Part model, mm, in its own coordinate system. A direction names the side the tool comes from. Coordinates: 2 decimals unless noted, no trailing zeros. Order: outer loops, then holes, each group sorted by start corner. A loop starts at its lowest first (then second) coordinate and runs counter-clockwise, first axis right, second up.
from build123d import *

# Parameters (mm, degrees)
CROQUIS1_R              = 20.65
CROQUIS1_R_2            = 1.5
SALIENTE_EXTRUIR1_DEPTH = 5
SALIENTE_EXTRUIR2_DEPTH = 20
CROQUIS3_R              = 1.5
CORTAR_EXTRUIR1_DEPTH   = 20
CROQUIS4_R              = 2
CORTAR_EXTRUIR2_DEPTH   = 166.327956902
CHAFL_N1_SIZE           = 15
CROQUIS5_R              = 7
CROQUIS5_R_2            = 2
CORTAR_EXTRUIR3_DEPTH   = 30
CORTAR_EXTRUIR4_START   = 30
CROQUIS6_R              = 6.5
CROQUIS6_R_2            = 1.5
CORTAR_EXTRUIR4_DEPTH   = 30


with BuildPart() as part:
    # Croquis1 → Saliente-Extruir1 (new, symmetric)
    with BuildSketch(Plane(origin=(0, 0, 0), x_dir=(0, 0, -1), z_dir=(1, 0, 0))):
        with BuildLine():
            Line((-109.696551146, -120), (109.696551146, -120))
            Line((109.696551146, -120), (30.310889132, 17.5))
            ThreePointArc((30.310889132, 17.5), (0, 35), (-30.310889132, 17.5))
            Line((-30.310889132, 17.5), (-109.696551146, -120))
        make_face()
        Circle(CROQUIS1_R, mode=Mode.SUBTRACT)
        with Locations((-30, 0)):
            Circle(CROQUIS1_R_2, mode=Mode.SUBTRACT)
        with Locations((30, 0)):
            Circle(CROQUIS1_R_2, mode=Mode.SUBTRACT)
    extrude(amount=SALIENTE_EXTRUIR1_DEPTH, both=True)

    # Croquis2 → Saliente-Extruir2 (add)
    with BuildSketch(Plane.ZY.offset(5)):
        Polygon((-109.696551146, -120), (-103.923048454, -110), (103.923048454, -110), (109.696551146, -120), align=None)
    extrude(amount=SALIENTE_EXTRUIR2_DEPTH)

    # Croquis3 → Cortar-Extruir1 (cut)
    with BuildSketch(Plane(origin=(0, -110, 0), x_dir=(1, 0, 0), z_dir=(0, 1, 0))):
        with Locations(Location((-15, 60, 0), (0, 0, 270))):
            Circle(CROQUIS3_R)
        with Locations(Location((-15, -60, 0), (0, 0, 270))):
            Circle(CROQUIS3_R)
        with Locations(Location((-15, 0, 0), (0, 0, 270))):
            Circle(CROQUIS3_R)
    extrude(amount=-CORTAR_EXTRUIR1_DEPTH, mode=Mode.SUBTRACT)

    # Croquis4 → Cortar-Extruir2 (cut, through all)
    with BuildSketch(Plane(origin=(5, 0, 0), x_dir=(0, 0, -1), z_dir=(1, 0, 0))):
        with Locations((-40, -100)):
            Circle(CROQUIS4_R)
        with Locations((40, -100)):
            Circle(CROQUIS4_R)
    extrude(amount=-CORTAR_EXTRUIR2_DEPTH, mode=Mode.SUBTRACT)

    # Chaflán1
    # the kernel refuses this chamfer: 15 mm, written as the material it adds along each edge
    with BuildSketch(Plane(origin=(-5, -110, -142.498293274), x_dir=(0.02749587661058636, 0.9996219169112966, 0), z_dir=(0, 0, 1))) as chafl_n1_piece_1_section:
        Polygon((CHAFL_N1_SIZE * 0.999621916911, CHAFL_N1_SIZE * 0.0274958766106), (-CHAFL_N1_SIZE * 0.0274958766106, CHAFL_N1_SIZE * 0.999621916911), (0, 0), align=None)
    chafl_n1_piece_1 = extrude(amount=284.996586547, mode=Mode.PRIVATE)
    chafl_n1_piece_1 = split(chafl_n1_piece_1, bisect_by=Plane(origin=(-9.982063802, -61.362690363, 75.842284643), z_dir=(0, -0.500000000000004, -0.8660254037844364)), keep=Keep.TOP, mode=Mode.PRIVATE)
    chafl_n1_piece_1 = split(chafl_n1_piece_1, bisect_by=Plane(origin=(-9.982063802, -61.362690271, -75.84228459), z_dir=(0, -0.4999999999999981, 0.8660254037844397)), keep=Keep.TOP, mode=Mode.PRIVATE)
    chafl_n1_piece_1 = chafl_n1_piece_1 - Plane(origin=(-9.982063802, -100, 40), x_dir=(0, 0, -1), z_dir=(1, 0, 0)) * Cylinder(2, 630, mode=Mode.PRIVATE)
    chafl_n1_piece_1 = chafl_n1_piece_1 - Plane(origin=(-9.982063802, -100, -40), x_dir=(0, 0, -1), z_dir=(1, 0, 0)) * Cylinder(2, 630, mode=Mode.PRIVATE)
    chafl_n1_piece_1 = chafl_n1_piece_1 - Plane(origin=(-15, -105.150253756, -60), x_dir=(0, 0, 1), z_dir=(0, 1, 0)) * Cylinder(1.5, 630, mode=Mode.PRIVATE)
    chafl_n1_piece_1 = chafl_n1_piece_1 - Plane(origin=(-15, -105.150253756, 0), x_dir=(0, 0, 1), z_dir=(0, 1, 0)) * Cylinder(1.5, 630, mode=Mode.PRIVATE)
    chafl_n1_piece_1 = chafl_n1_piece_1 - Plane(origin=(-15, -105.150253756, 60), x_dir=(0, 0, 1), z_dir=(0, 1, 0)) * Cylinder(1.5, 630, mode=Mode.PRIVATE)
    add(chafl_n1_piece_1)

    # Croquis5 → Cortar-Extruir3 (cut)
    # profile 1 of 2: a face of its own
    with BuildSketch(Plane.ZY.offset(5)):
        with Locations((-40, -100)):
            Circle(CROQUIS5_R)
        with Locations(Location((-40, -100, 0), (0, 0, 180))):
            Circle(CROQUIS5_R_2, mode=Mode.SUBTRACT)
    # profile 2 of 2: a face of its own
    with BuildSketch(Plane.ZY.offset(5)):
        with Locations((40, -100)):
            Circle(CROQUIS5_R)
        with Locations(Location((40, -100, 0), (0, 0, 180))):
            Circle(CROQUIS5_R_2, mode=Mode.SUBTRACT)
    extrude(amount=CORTAR_EXTRUIR3_DEPTH, mode=Mode.SUBTRACT)

    # Croquis6 → Cortar-Extruir4 (cut)
    # profile 1 of 3: a face of its own
    with BuildSketch(Plane(origin=(0, -110, 0), x_dir=(1, 0, 0), z_dir=(0, 1, 0)).offset(CORTAR_EXTRUIR4_START)):
        with Locations((-15, 60)):
            Circle(CROQUIS6_R)
        with Locations(Location((-15, 60, 0), (0, 0, 270))):
            Circle(CROQUIS6_R_2, mode=Mode.SUBTRACT)
    # profile 2 of 3: a face of its own
    with BuildSketch(Plane(origin=(0, -110, 0), x_dir=(1, 0, 0), z_dir=(0, 1, 0)).offset(CORTAR_EXTRUIR4_START)):
        with Locations((-15, 0)):
            Circle(CROQUIS6_R)
        with Locations(Location((-15, 0, 0), (0, 0, 270))):
            Circle(CROQUIS6_R_2, mode=Mode.SUBTRACT)
    # profile 3 of 3: a face of its own
    with BuildSketch(Plane(origin=(0, -110, 0), x_dir=(1, 0, 0), z_dir=(0, 1, 0)).offset(CORTAR_EXTRUIR4_START)):
        with Locations((-15, -60)):
            Circle(CROQUIS6_R)
        with Locations(Location((-15, -60, 0), (0, 0, 270))):
            Circle(CROQUIS6_R_2, mode=Mode.SUBTRACT)
    extrude(amount=-CORTAR_EXTRUIR4_DEPTH, mode=Mode.SUBTRACT)


solid = part.part
Q1. Cut at C-C on x = -22.5. Write the cut outline in (y, z).
Results list:
outline: (-120, -109.7) - (-110, -103.92) - (-110, 103.92) - (-120, 109.7) - close
Q2. Which spindle directions (+Z, -Z, +X, -X, +Y, -Y) get a long thin tool onto all of the face, cutting with end or side? Do faces 1 (the face through (-10, -107, 40)), 2 (the face through (-8.504, -105.447, 60.223)), 3 (the face through (-10, -120, 2)). Say none if no direction does.
Results list:
face 1: -X
face 2: +Y
face 3: +Z, -Z, +X, -X, -Y
Q3. Wall check: line 1 along Z through (x, y) = (-15, -105.75); line 2 along Z through (x, y) = (-2.5, -100); line 3 along X through (y, z) = (-113.5, 0). Give the ranges that are in metal, low to high.
Results list:
line 1: z = -101.47 to -66.5, -53.5 to -43.99, -36.01 to -6.5, 6.5 to 36.01, 43.99 to 53.5, 66.5 to 101.47
line 2: z = -98.15 to -42, -38 to 38, 42 to 98.15
line 3: x = -25 to -16.5, -13.5 to 5
Q4. Pin check, flat tips, straight feed: pin 1 Ø12 at (x, z) = (-7.5, 51) entering from +Y; pin 2 Ø12 at (x, y) = (-1, 13) entering from +Z; pin 3 Ø10.5 at (x, z) = (-15, -60) entering from +Y. Stop position of each tip, or through.
Results list:
pin 1: stops at y = -8.89
pin 2: stops at z = 36.37
pin 3: stops at y = -110
Q5. Mould opens along Z. For faces 4 (the face through (-10, -107, -40)), 5 (the face through (0.07, 34.996, -0.513)), 6 (the face through (-7, -97, -1)) say: pulls with the +Z half, pulls with the -Z half, needs draft (parallel to the pull), parting line crosses it, or undercut.
Results list:
face 4: undercut
face 5: parting line crosses it
face 6: needs draft
Q6. Cut at A-A on x = 1.5. Write the cut outline in (y, z).
Results list:
outline: (-120, -109.7) - (17.5, -30.31) arc R35 ccw to (17.5, 30.31) - (-120, 109.7) - close; hole circle Ø4 at (-100, -40); hole circle Ø4 at (-100, 40); hole circle Ø41.3 at (0, 0); hole circle Ø3 at (0, -30); hole circle Ø3 at (0, 30)
Q7. Cut at B-B on y = -88. Write the cut outline in (x, z).
Results list:
outline: (-5, -91.22) - (5, -91.22) - (5, 91.22) - (-5, 91.22) - close
